from build123d import *

# Parameters (mm, degrees)
BOSS_EXTRUDE2_DEPTH = 100
SKETCH3_W           = 11
SKETCH3_H           = 22
SKETCH4_R           = 1
CUT_EXTRUDE1_DEPTH  = 2
SKETCH5_R           = 1
CUT_EXTRUDE2_DEPTH  = 2
CIRPATTERN1_COUNT   = 4
SKETCH6_W           = 10
SKETCH6_H           = 190
BOSS_EXTRUDE4_DEPTH = 115
SKETCH10_W          = 10
SKETCH10_H          = 190
SKETCH11_R          = 1
CUT_EXTRUDE3_DEPTH  = 2
SKETCH8_R           = 2.5
SKETCH8_W           = 20
SKETCH8_H           = 5
CUT_EXTRUDE4_DEPTH  = 10
SKETCH12_R          = 75
CUT_EXTRUDE5_DEPTH  = 30


with BuildPart() as part:
    # Sketch1 → Boss-Extrude2 (new body)
    with BuildSketch(Plane(origin=(0, 0, 0), x_dir=(1, 0, 0), z_dir=(0, 1, 0))):
        with BuildLine():
            ThreePointArc((75, 0), (53.033008589, 53.033008589), (0, 75))
            Line((0, 75), (0, -75))
            ThreePointArc((0, -75), (53.033008589, -53.033008589), (75, 0))
        make_face()
    extrude(amount=BOSS_EXTRUDE2_DEPTH)

    # Sketch3 → Cut-Revolve3 (revolve, cut)
    with BuildSketch(Plane(origin=(0, 0, 0), x_dir=(-1, 0, 0), z_dir=(0, -1, 0))):
        with Locations((-59.5, 11)):
            Rectangle(SKETCH3_W, SKETCH3_H)
    cut_revolve3 = revolve(axis=Axis((0, 0, 0), (1, 0, 0)), mode=Mode.SUBTRACT)

    # Sketch4 → Cut-Extrude1 (cut)
    with BuildSketch(Plane.ZY.offset(-65)):
        Circle(SKETCH4_R)
    cut_extrude1 = extrude(amount=-CUT_EXTRUDE1_DEPTH, mode=Mode.SUBTRACT)

    # Sketch5 → Cut-Extrude2 (cut)
    with BuildSketch(Plane(origin=(54, 0, 0), x_dir=(0, 0, -1), z_dir=(1, 0, 0))):
        Circle(SKETCH5_R)
    cut_extrude2 = extrude(amount=-CUT_EXTRUDE2_DEPTH, mode=Mode.SUBTRACT)

    # CirPattern1: Cut-Revolve3, Cut-Extrude1, Cut-Extrude2 ×4 about axis
    cirpattern1_axis = Axis((0, 0, 0), (0, 1, 0))
    add([cut_revolve3.rotate(cirpattern1_axis, i * 360 / CIRPATTERN1_COUNT) for i in range(1, CIRPATTERN1_COUNT)], mode=Mode.SUBTRACT)
    add([cut_extrude1.rotate(cirpattern1_axis, i * 360 / CIRPATTERN1_COUNT) for i in range(1, CIRPATTERN1_COUNT)], mode=Mode.SUBTRACT)
    add([cut_extrude2.rotate(cirpattern1_axis, i * 360 / CIRPATTERN1_COUNT) for i in range(1, CIRPATTERN1_COUNT)], mode=Mode.SUBTRACT)

    # Sketch6 → Boss-Extrude4 (add)
    with BuildSketch(Plane(origin=(0, 100, 0), x_dir=(1, 0, 0), z_dir=(0, 1, 0))):
        with Locations((5, -95)):
            Rectangle(SKETCH6_W, SKETCH6_H)
    extrude(amount=BOSS_EXTRUDE4_DEPTH)

    # Sketch10 → Cut-Revolve4 (revolve, cut)
    with BuildSketch(Plane(origin=(0, 215, 0), x_dir=(1, 0, 0), z_dir=(0, 1, 0))):
        with Locations((5, -95)):
            Rectangle(SKETCH10_W, SKETCH10_H)
    revolve(axis=Axis((10, 215, 0), (-1, 0, 0)), mode=Mode.SUBTRACT)


with BuildPart() as cut_revolve4_kept_piece:
    # of the separate pieces the step leaves, the one the design keeps (cut_revolve4_pieces_kept)
    add(part.part.solids().sort_by_distance((0, 0, 75))[0])

    # Sketch11 → Cut-Extrude3 (cut)
    with BuildSketch(Plane.ZY.offset(-10)):
        with Locations((-0.669656263, 47.5)):
            Circle(SKETCH11_R)
        with Locations((-65.669656263, 60.5)):
            Circle(SKETCH11_R)
        with Locations((64.330343737, 60.5)):
            Circle(SKETCH11_R)
    extrude(amount=-CUT_EXTRUDE3_DEPTH, mode=Mode.SUBTRACT)

    # Sketch8 → Cut-Extrude4 (cut)
    with BuildSketch(Plane.ZY):
        with Locations((-70, 10)):
            Circle(SKETCH8_R)
        with Locations(Location((70, 10, 0), (0, 0, 180))):
            Circle(SKETCH8_R)
        with Locations((-30, 2.5)):
            Rectangle(SKETCH8_W, SKETCH8_H)
        with Locations((30, 2.5)):
            Rectangle(SKETCH8_W, SKETCH8_H)
    extrude(amount=-CUT_EXTRUDE4_DEPTH, mode=Mode.SUBTRACT)

    # Sketch12 → Cut-Extrude5 (cut)
    with BuildSketch(Plane(origin=(0, 100, 0), x_dir=(1, 0, 0), z_dir=(0, 1, 0))):
        Circle(SKETCH12_R)
    extrude(amount=-CUT_EXTRUDE5_DEPTH, mode=Mode.SUBTRACT)


solid = cut_revolve4_kept_piece.part
CAD build for the part. Positions are in the model's coordinates, mm. A direction names the side the tool comes from. Round coordinates to 2 decimals unless told otherwise and drop trailing zeros. Order: outer loops, then holes, each group sorted by start corner. A loop starts at its lowest first (then second) coordinate and runs counter-clockwise, first axis right, second up. Notation, with made-up numbers: (87.5, 78) -> (106.5, 78) arc R24 ccw to (106.5, 111) -> close; hole circle Ø1 at (-29.5, -12.5). An arc over 180 degrees is marked (long way). Write each question's results on one line, items separated by ' | '.
1. Cut at D-D (x = 49.5). Give the cut face in (y, z).
Findings below:
outline: (0, -56.34) -> (70, -56.34) -> (70, 56.34) -> (0, 56.34) -> close
2. Cut at B-B (z = -38.5). Give the cut face in (x, y).
Findings below:
outline: (0, 5) -> (10, 5) -> (10, 0) -> (64.36, 0) -> (64.36, 70) -> (10, 70) -> (10, 28.94) -> (0, 28.94) -> close
3. Cut at A-A (y = 10). Give the cut face in (x, z), plus the area to 3 significant figures.
Findings below:
outline: (0, -75) arc R75 ccw to (0, 75) -> (0, 72.5) -> (10, 72.5) -> (10, 67.5) -> (0, 67.5) -> (0, 65) -> (19.6, 65) -> (19.6, 54) -> (0, 54) -> (0, -54) -> (19.6, -54) -> (19.6, -65) -> (0, -65) -> (0, -67.5) -> (10, -67.5) -> (10, -72.5) -> (0, -72.5) -> close; hole (54, -19.6) -> (65, -19.6) -> (65, 19.6) -> (54, 19.6) -> close | area: 7,870 mm²
4. Pull direction Y, two halves, no side cores. Call faces 1 (the face through (9, 9, 54)), 2 (the face through (10, 10, 70)), 3 (the face through (5, 5, 30)): pulls with the +Y half, pulls with the -Y half, needs draft (parallel to the pull), parting line crosses it, or undercut.
Findings below:
face 1: needs draft | face 2: undercut | face 3: pulls with the -Y half
5. 3-axis set-ups, long thin cutter, end or side, ignore diameter. For faces 4 (the face through (8, 9, -65)), 5 (the face through (10, 10, -70)), 6 (the face through (5.07, 25.003, -1.079)): which of +Z, -Z, +X, -X, +Y, -Y reach the whole face in a straight line?
Findings below:
face 4: -X, -Y | face 5: -X | face 6: -X, +Y
6. Wall check: line 1 along Y through (x, z) = (4.75, -70); line 2 along X through (y, z) = (3, -9.5); line 3 along X through (y, z) = (55, 59). Give the ranges that are in metal, low to high. Write a range as [from, to].
Findings below:
line 1: y = [0, 7.5], [12.5, 38.36] | line 2: x = [0, 54], [65, 74.4] | line 3: x = [10, 46.3]
7. Cut at C-C (y = 54.5). Give the cut face in (x, z).
Findings below:
outline: (10, -74.33) arc R75 ccw to (10, 74.33) -> close
8. Flat gauge pins, fed straight in: P1, Ø6, axis at x = 25.5, y = 8.5, coming from the +Z side; P2, Ø10, axis at x = 29.5, y = 56, coming from the +Z side; P3, Ø12, axis at y = 16, z = -31, coming from the -X side; P4, Ø1.2, axis at y = 60.5, z = -65.67, coming from the -X side. Where does each tip first touch, or does it go through?
Findings below:
P1: stops at z = 71.55 | P2: stops at z = 70.89 | P3: stops at x = 0 | P4: stops at x = 12
